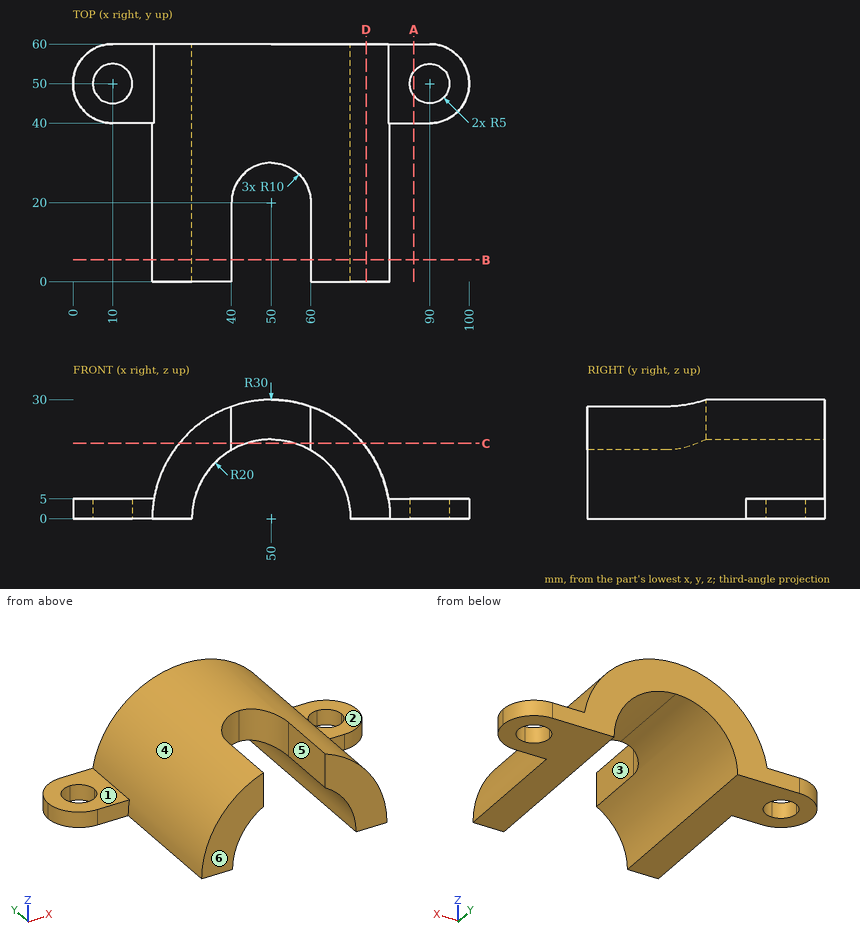
Could you check a few things on this drawing? It's one solid part, dimensions in mm from its lowest x, y, z. A direction names the side the tool comes from. Coordinates: 2 decimals unless noted, no trailing zeros. Order: outer loops, then holes, each group sorted by start corner. A loop starts at its lowest first (then second) coordinate and runs counter-clockwise, first axis right, second up. Notation, with made-up numbers: M 64,58 L 117,58 A15 cw 117,62 Z; hole C 13.25,22.25 d10. An arc over 180 degrees is marked long. Use a Markdown table: item, result. Add a question column.
Q1. I want a section at D-D on x = 74. List the corners of the cut face in (y, z) for me, then the cut area to 3 significant figures.
Q2. I want a section at A-A on x = 86. List the corners of the cut face in (y, z) for me, then the cut area to 3 significant figures.
Q3. We'd pull the mould along X, two halves only. Please class the marked faces 4, 5 and 6: pulls with the +X half, pulls with the -X half, needs draft (parallel to the pull), parting line crosses it, or undercut.
Q4. If I drill on L1, parallel to X at y = 25.5, z = 9.5; L2, parallel to Z at x = 16.5, y = 54; L3, parallel to X at y = 8, z = 15, over which ranges is the centre line in solid material (lowest first)?
Q5. I'm going to push flat-ended pins straight in: pin 1 (1 mm diameter, centred on y = 52.5, z = 14.5, fed in from +X); pin 2 (3 mm diameter, centred on y = 23, z = 23.5, fed in from -X); pin 3 (2 mm diameter, centred on x = 75, y = 31.5, fed in from +Z). Where does each tip first touch, or does it pass through?
Q6. Which directions (+Z, -Z, +X, -X, +Y, -Y) give clear straight access to the entire face, cutting with the end or side of a thin tool? Please do the marked faces 1, 2 and 3.
Q7. I want a section at B-B on y = 5.5. List the corners of the cut face in (x, z) for me, then the cut area to 3 significant figures.
Q8. I want a section at C-C on z = 19. List the corners of the cut face in (x, y) for me (3 decimals), then the cut area to 3 significant figures.
Checked values:
| question | item | result |
|---|---|---|
| 1 | outline | M 0,0 L 60,0 L 60,18 L 0,18 Z |
| 1 | area | 1,080 mm² |
| 2 | outline | M 40,0 L 47,0 L 47,5 L 40,5 Z; M 53,0 L 60,0 L 60,5 L 53,5 Z |
| 2 | area | 70.0 mm² |
| 3 | face 4 | parting line crosses it |
| 3 | face 5 | undercut |
| 3 | face 6 | needs draft |
| 4 | L1 | 21.54 to 32.4, 67.6 to 78.46 |
| 4 | L2 | 0 to 5 |
| 4 | L3 | 24.02 to 36.77, 63.23 to 75.98 |
| 5 | pin 1 | x = 76.53 |
| 5 | pin 2 | x = 29.6 |
| 5 | pin 3 | z = 18 |
| 6 | face 1 | +Z, -X, +Y, -Y |
| 6 | face 2 | +Z, +X, +Y, -Y |
| 6 | face 3 | +Z, -Z, -Y |
| 7 | outline | M 20,0 L 30,0 A20 cw 40,17.32 L 40,28.28 A30 ccw Z; M 60,17.32 A20 cw 70,0 L 80,0 A30 ccw 60,28.28 Z |
| 7 | area | 579 mm² |
| 8 | outline | M 26.784,0 L 40,0 L 40,20 A10 cw 43.755,27.81 L 43.755,60 L 26.784,60 Z; M 56.245,27.81 A10 cw 60,20 L 60,0 L 73.216,0 L 73.216,60 L 56.245,60 Z |
| 8 | area | 1,850 mm² |
